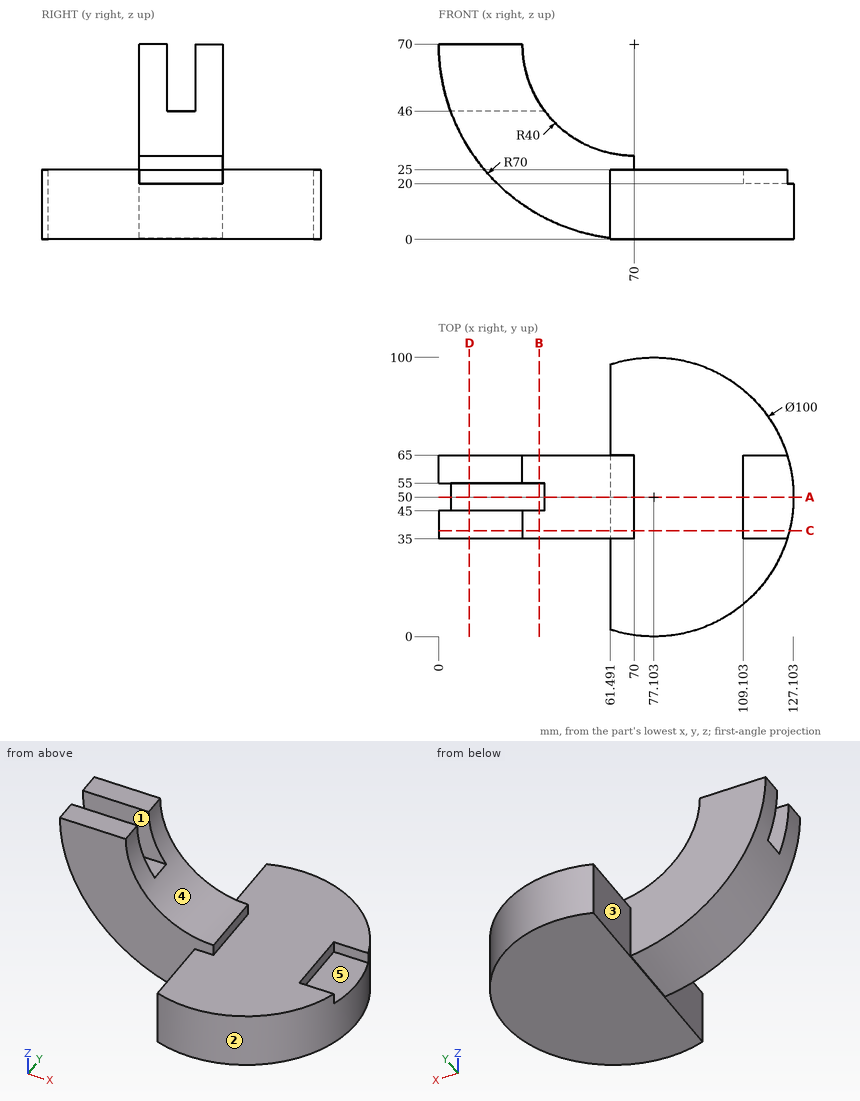
Part print with two shaded views. Sizes in mm from the minimum x, y, z corner. A direction names the side the tool comes from. Give positions to 0.01 mm unless a question says otherwise; leave off trailing zeros. Loops run counter-clockwise (first coordinate to the right, second up) from the corner with the lowest first, then second, coordinate; pieces in that order, holes last. Notation, with made-up numbers: (75, 49) -> (111, 49) arc R22 ccw to (111, 67) -> close; hole circle Ø3 at (-26.75, 63). An arc over 180 degrees is marked (long way). One line per question, with ' | ' between items.
Q1. Tool access for the marked faces 4 and 5: list every direction of +Z, -Z, +X, -X, +Y, -Y with a clear straight run to the whole face (end or side of a thin tool).
Filled sheet:
face 4: +Z, +X, +Y, -Y | face 5: +Z, +X
Q2. Cut at C-C, the plane y = 38. Write the cut outline in (x, z), plus the area to 3 significant figures.
Filled sheet:
outline: (0, 70) arc R70 ccw to (61.49, 0.52) -> (61.49, 0) -> (125.64, 0) -> (125.64, 20) -> (109.1, 20) -> (109.1, 25) -> (70, 25) -> (70, 30) arc R40 cw to (30, 70) -> close | area: 3,900 mm²
Q3. Drop flat-ended pins along their axis: pin 1 (10 mm diameter, centred on y = 28, z = 14.5, fed in from -X); pin 2 (5.5 mm diameter, centred on y = 46, z = 23.5, fed in from +X); pin 3 (19 mm diameter, centred on x = 16.5, z = 60.5, fed in from +Y). Give the stop position or say it passes through.
Filled sheet:
pin 1: stops at x = 61.49 | pin 2: stops at x = 109.1 | pin 3: stops at y = 65
Q4. Cut at A-A, the plane y = 50. Write the cut outline in (x, z), plus the area to 3 significant figures.
Filled sheet:
outline: (4.24, 46) arc R70 ccw to (61.49, 0.52) -> (61.49, 0) -> (127.1, 0) -> (127.1, 20) -> (109.1, 20) -> (109.1, 25) -> (70, 25) -> (70, 30) arc R40 cw to (38, 46) -> close | area: 3,180 mm²
Q5. Drill centre lines: line 1 along Y through (x, z) = (31, 31.5); line 2 along Z through (x, y) = (93, 62); line 3 along X through (y, z) = (44.5, 36) (1 decimal). Where is each one in solid material? Low to high. Write a range as [from, to].
Filled sheet:
line 1: y = [35, 65] | line 2: z = [0, 25] | line 3: x = [8.8, 48.9]
Q6. Cut at B-B, the plane x = 36. Write the cut outline in (y, z).
Filled sheet:
outline: (35, 8.81) -> (65, 8.81) -> (65, 48.93) -> (55, 48.93) -> (55, 46) -> (45, 46) -> (45, 48.93) -> (35, 48.93) -> close
Q7. Cut at D-D, the plane x = 11. Write the cut outline in (y, z).
Filled sheet:
outline: (35, 32.33) -> (65, 32.33) -> (65, 70) -> (55, 70) -> (55, 46) -> (45, 46) -> (45, 70) -> (35, 70) -> close
Q8. Pull direction Y, two halves, no side cores. Call the marked faces 1, 2 and 3: pulls with the +Y half, pulls with the -Y half, needs draft (parallel to the pull), parting line crosses it, or undercut.
Filled sheet:
face 1: undercut | face 2: parting line crosses it | face 3: needs draft
